from build123d import *

# Parameters (mm, degrees)
F0_W     = 20
F0_H     = 30
F1_DEPTH = 10
F2_W     = 10.8
F2_H     = 3.1583849106
F3_DEPTH = 5.4
F4_DEPTH = 8.1
F5_R     = 2.5
F6_DEPTH = 20


with BuildPart() as f1:
    # F0 (on Top) → F1 (new body)
    with BuildSketch(Plane.XY):
        Rectangle(F0_W, F0_H)
    extrude(amount=F1_DEPTH)

    # F2 (on face) → F3 (cut)
    with BuildSketch(Plane(origin=(-10, 0, 0), x_dir=(0, -1, 0), z_dir=(-1, 0, 0))):
        with Locations((-3.6, 1.5791924553)):
            Rectangle(F2_W, F2_H)
    extrude(amount=-F3_DEPTH, mode=Mode.SUBTRACT)

    # F2 (on face) → F4 (cut)
    with BuildSketch(Plane(origin=(-10, 0, 0), x_dir=(0, -1, 0), z_dir=(-1, 0, 0))):
        Polygon((-12.7, 3.1583849106), (-9, 3.1583849106), (1.8, 3.1583849106), (5.5, 3.1583849106), (5.5, 6.8666899811), (-12.7, 6.8666899811), align=None)
    extrude(amount=-F4_DEPTH, mode=Mode.SUBTRACT)

    # F5 (on face) → F6 (cut)
    with BuildSketch(Plane(origin=(-10, 0, 0), x_dir=(0, -1, 0), z_dir=(-1, 0, 0))):
        with Locations((10.7573593129, 5.7)):
            Circle(F5_R)
    extrude(amount=-F6_DEPTH, mode=Mode.SUBTRACT)


solid = f1.part
Geometry: final body of the model. Coordinates: model frame, mm. A direction names the side the tool comes from. Round coordinates to 2 decimals unless told otherwise and drop trailing zeros. Loops run counter-clockwise (first coordinate to the right, second up) from the corner with the lowest first, then second, coordinate; pieces in that order, holes last.
Q1. Pull-direction query (Z, two-part tool) for faces 4 (the flat face through (0, 0, 0)), 5 (the flat face through (0, 0, 10)), 6 (the flat face through (-7, 9, 2)), 7 (the flat face through (-4, 4, 3.158)); classes: released by +Z, released by -Z, zero draft, split by the parting line, or undercut.
Q2. Material intervals for L1, parallel to Z at x = -3.25, y = -1; L2, parallel to Y at x = -8.25, z = 3.5; L3, parallel to Y at x = -9, z = 4, sorted ascending.
Q3. Section B-B on y = -0.75. Return loops of the section in (x, z).
Q4. Section D-D on y = -9.25. Return loops of the section in (x, z), plus the area to 3 significant figures.
Q5. Pin query (flat end, axial travel): P1, Ø1.6, axis at y = 1.5, z = 1.5, coming from the -X side; P2, Ø4, axis at y = -10.76, z = 5.7, coming from the +X side (3 decimals); P3, Ø3, axis at y = 4.5, z = 5, coming from the -X side. Return the tip coordinate at first contact, or that it passes through.
Q6. Section A-A on z = 5.7. Return loops of the section in (x, y), plus the area to 3 significant figures.
Q7. Access query for faces 1 (the flat face through (-7, -1.8, 2)), 2 (the cylindrical face through (-0.14, -10.22, 3.26)), 3 (the flat face through (-6, -5.5, 5)). Directions: +Z, -Z, +X, -X, +Y, -Y. A direction counts if a zero-diameter tool reaches every point of the face in a straight line with its end or side. Return the directions, or none.
Q8. Section C-C on x = -7.5. Return loops of the section in (y, z), plus the area to 3 significant figures.
Evaluation:
1. face 4: released by -Z
1. face 5: released by +Z
1. face 6: zero draft
1. face 7: undercut
2. L1: z = 0 to 3.16, 6.87 to 10
2. L2: y = -15 to -11.94, -9.57 to -5.5, 12.7 to 15
2. L3: y = -15 to -12.59, -8.92 to -5.5, 12.7 to 15
3. outline: (-10, 6.87) - (-1.9, 6.87) - (-1.9, 3.16) - (-4.6, 3.16) - (-4.6, 0) - (10, 0) - (10, 10) - (-10, 10) - close
4. outline: (-10, 0) - (10, 0) - (10, 3.71) - (-10, 3.71) - close; (-10, 7.69) - (10, 7.69) - (10, 10) - (-10, 10) - close
4. area: 120 mm2
5. P1: stops at x = -4.6
5. P2: passes through
5. P3: stops at x = -1.9
6. outline: (-10, -15) - (10, -15) - (10, -13.26) - (-10, -13.26) - close; (-10, -8.26) - (10, -8.26) - (10, 15) - (-10, 15) - (-10, 12.7) - (-1.9, 12.7) - (-1.9, -5.5) - (-10, -5.5) - close
6. area: 353 mm2
7. face 1: -Z, -X
7. face 2: +X, -X
7. face 3: -X
8. outline: (-15, 0) - (-1.8, 0) - (-1.8, 3.16) - (-5.5, 3.16) - (-5.5, 6.87) - (12.7, 6.87) - (12.7, 3.16) - (9, 3.16) - (9, 0) - (15, 0) - (15, 10) - (-15, 10) - close; hole circle Ø5 at (-10.76, 5.7)
8. area: 179 mm2
